Could you check a few things on this model? Use its own coordinates, in mm. Coordinates: 2 decimals unless noted, no trailing zeros. Order: outer loops, then holes, each group sorted by start corner. A loop starts at its lowest first (then second) coordinate and runs counter-clockwise, first axis right, second up. Notation, with made-up numbers: (-33.5, 55.25) -> (-12.5, 55.25) arc R23 ccw to (-12.5, 75.25) -> close; hole circle Ø5 at (13, -10). An arc over 180 degrees is marked (long way). Put each result on its own line as item: value. Start each with the question number.
Q1. If we section it at C-C (x = 79.5): Please give me the cut outline in (y, z).
Q2. Will these pins go through, and if not, where does the flat tip stop? pin 1 (10 mm diameter, centred on x = 127, y = -50.8, fed in from -Z); pin 2 (3 mm diameter, centred on x = 63.5, y = -50.8, fed in from -Z); pin 3 (2 mm diameter, centred on x = 43, z = 1, fed in from +Y) (3 decimals).
Q3. We'd pull the mould along Y, two halves only. Please class faces 1 (the face through (10.562, -39.276, 2.421)), 2 (the face through (46, -43, 0)), 3 (the face through (128.707, -48.123, 2.421)), 4 (the face through (-0.52, -2.33, 2.42)): +Y half, -Y half, draft (parallel to the pull), parting line (faces both ways), or undercut.
Q4. If we section it at D-D (y = -34.5): Please give me the cut outline in (x, z), and give its area (3 significant figures).
Q5. If we section it at B-B (x = 107.95): Please give me the cut outline in (y, z).
Q6. Please list where these lines run through material, in increasing order: line 1 along X through (y, z) = (-51, 3.9); line 2 along X through (y, z) = (-49, 1.15); line 3 along Y through (x, z) = (0.5, 3.8).
from build123d import *

# Parameters (mm, degrees)
BOSS_EXTRUDE1_DEPTH = 4.7752
FILLET1_R           = 4.7752
SKETCH2_R           = 2.3876
CUT_EXTRUDE1_DEPTH  = 151.645704088
SKETCH3_R           = 3.175
CUT_EXTRUDE2_DEPTH  = 4.7752


with BuildPart() as part:
    # Sketch1 → Boss-Extrude1 (new body)
    with BuildSketch(Plane.XY):
        with BuildLine():
            ThreePointArc((7.9502, 0), (0, 7.9502), (-7.9502, 0))
            Line((-7.9502, 0), (-9.506710526, -50.210016974))
            Line((-9.506710526, -50.210016974), (-9.525, -50.8))
            ThreePointArc((-9.525, -50.8), (-6.735192091, -57.535192091), (0, -60.325))
            Line((0, -60.325), (62.233167082, -63.436658354))
            Line((62.233167082, -63.436658354), (63.5, -63.5))
            Line((63.5, -63.5), (64.766832918, -63.436658354))
            Line((64.766832918, -63.436658354), (127, -60.325))
            ThreePointArc((127, -60.325), (136.525, -50.8), (127, -41.275))
            Line((127, -41.275), (64.766832918, -38.163341646))
            Line((64.766832918, -38.163341646), (63.5, -38.1))
            Line((63.5, -38.1), (62.233167082, -38.163341646))
            Line((62.233167082, -38.163341646), (9.215441066, -40.814227947))
            Line((9.215441066, -40.814227947), (7.9502, 0))
        make_face()
        with BuildLine():
            Line((9.525, -50.8), (9.506710526, -50.210016974))
            ThreePointArc((9.506710526, -50.210016974), (9.520426534, -50.504866777), (9.525, -50.8))
        make_face(mode=Mode.SUBTRACT)
    extrude(amount=BOSS_EXTRUDE1_DEPTH)

    # Fillet1
    fillet1_edges = [part.edges().sort_by_distance(p)[0] for p in [
        (9.215441066, -40.814227947, 2.3876),
    ]]
    fillet(fillet1_edges, radius=FILLET1_R)

    # Sketch2 → Cut-Extrude1 (cut, through all)
    with BuildSketch(Plane.XY.offset(4.7752)):
        Circle(SKETCH2_R)
        with Locations((0, -50.8)):
            Circle(SKETCH2_R)
        with Locations((63.5, -50.8)):
            Circle(SKETCH2_R)
        with Locations((107.95, -50.8)):
            Circle(SKETCH2_R)
    extrude(amount=-CUT_EXTRUDE1_DEPTH, mode=Mode.SUBTRACT)

    # Sketch3 → Cut-Extrude2 (cut)
    with BuildSketch(Plane.XY.offset(4.7752)):
        with Locations((127, -50.8)):
            Circle(SKETCH3_R)
    extrude(amount=-CUT_EXTRUDE2_DEPTH, mode=Mode.SUBTRACT)


solid = part.part
The answers:
1. outline: (-62.7, 0) -> (-38.9, 0) -> (-38.9, 4.78) -> (-62.7, 4.78) -> close
2. pin 1: z = 0
2. pin 2: through
2. pin 3: y = -39.075
3. face 1: +Y half
3. face 2: draft
3. face 3: undercut
3. face 4: undercut
4. outline: (-9.02, 0) -> (9.02, 0) -> (9.02, 4.78) -> (-9.02, 4.78) -> close
4. area: 86.1 mm^2
5. outline: (-61.28, 0) -> (-53.19, 0) -> (-53.19, 4.78) -> (-61.28, 4.78) -> close; (-48.41, 0) -> (-40.32, 0) -> (-40.32, 4.78) -> (-48.41, 4.78) -> close
6. line 1: -9.52 to -2.38, 2.38 to 61.12, 65.88 to 105.57, 110.33 to 123.83, 130.17 to 136.52
6. line 2: -9.47 to -1.57, 1.57 to 61.93, 65.07 to 106.38, 109.52 to 124.38, 129.62 to 136.35
6. line 3: -60.35 to -53.13, -48.47 to -2.33, 2.33 to 7.93
